Drawing for the job (mm, zero at the part's lowest x, y, z). A direction names the side the tool comes from. Round coordinates to 2 decimals unless told otherwise and drop trailing zeros. Loops run counter-clockwise (first coordinate to the right, second up) from the corner with the lowest first, then second, coordinate; pieces in that order, holes last. Notation, with made-up numbers: M -14.5,16.5 L 41.5,16.5 A25 cw 41.5,51.5 Z; hole C 6,15.5 d10. An arc over 180 degrees is marked long. Use a Markdown table: item, result. Add a question column.
Q1. Mould opens along Y. For the marked faces 1, 2, 3 and 4 say: +Y half, -Y half, draft (parallel to the pull), parting line (faces both ways), or undercut.
Q2. Cut at C-C (y = 18.5). Give the cut face in (x, z).
Q3. Probe line 1 (Y direction, x = 6.85, z = 0.6); line 2 (Z direction, x = 3, y = 13); line 3 (Z direction, x = 13, y = 24). List the from-to ranges inside material, lowest first. Write a range as from..to.
Q4. Tool access for the marked faces 5, 6 and 7: list every direction of +Z, -Z, +X, -X, +Y, -Y with a clear straight run to the whole face (end or side of a thin tool).
Q5. Cut at D-D (x = 11.25). Give the cut face in (y, z).
Q6. Pin check, flat tips, straight feed: pin 1 (2.5 mm diameter, centred on x = 6.85, y = 10.025, fed in from +Z); pin 2 (2 mm diameter, centred on y = 7, z = 7, fed in from +X); pin 3 (3 mm diameter, centred on x = 9, z = 5.5, fed in from +Y); pin 4 (4.5 mm diameter, centred on y = 20, z = 5.5, fed in from -X). Stop position of each tip, or through.
Q7. Cut at B-B (z = 5.75). Give the cut face in (x, y).
Q8. Cut at A-A (x = 6.85). Give the cut face in (y, z).
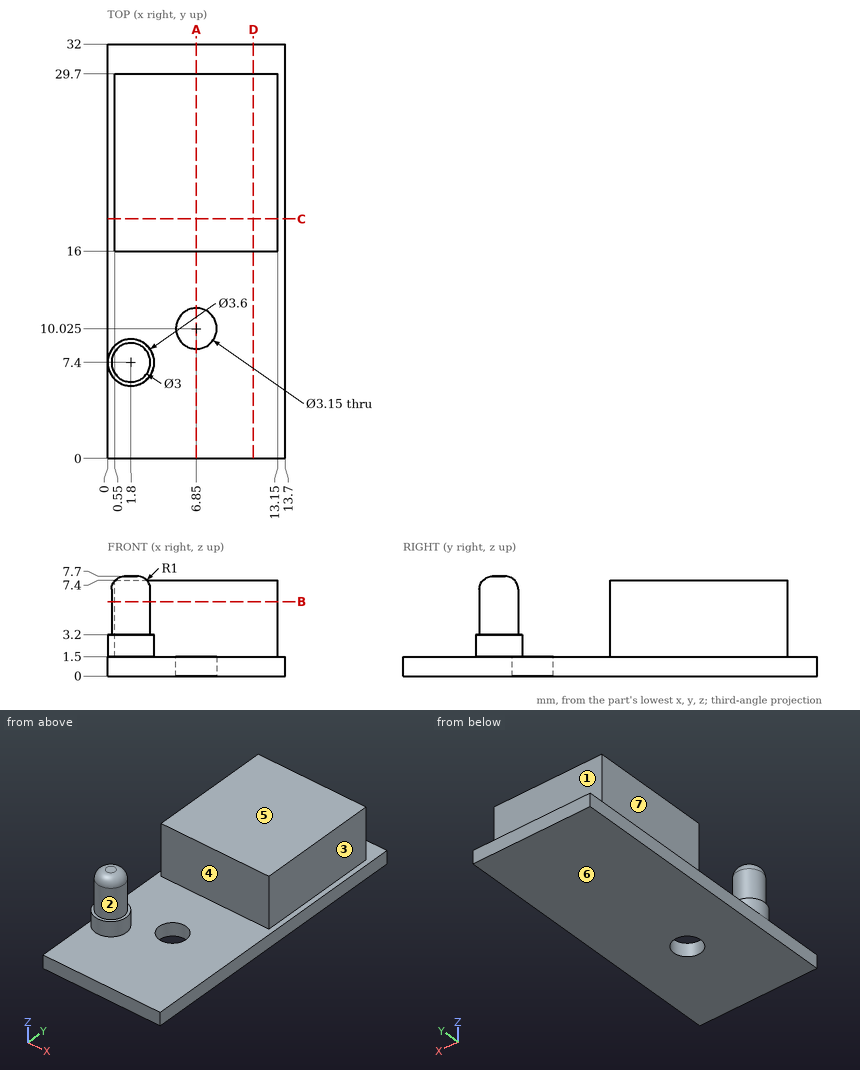
Checked values:
| question | item | result |
|---|---|---|
| 1 | face 1 | +Y half |
| 1 | face 2 | undercut |
| 1 | face 3 | draft |
| 1 | face 4 | undercut |
| 2 | outline | M 0,0 L 13.7,0 L 13.7,1.5 L 13.15,1.5 L 13.15,7.4 L 0.55,7.4 L 0.55,1.5 L 0,1.5 Z |
| 3 | line 1 | y = 0..8.45, 11.6..32 |
| 3 | line 2 | z = 0..1.5 |
| 3 | line 3 | z = 0..7.4 |
| 4 | face 5 | +Z, +X, -X, +Y |
| 4 | face 6 | -Z, +X, -X, +Y, -Y |
| 4 | face 7 | +Z, -X, +Y |
| 5 | outline | M 0,0 L 32,0 L 32,1.5 L 29.7,1.5 L 29.7,7.4 L 16,7.4 L 16,1.5 L 0,1.5 Z |
| 6 | pin 1 | passes through |
| 6 | pin 2 | stops at x = 3.3 |
| 6 | pin 3 | stops at y = 29.7 |
| 6 | pin 4 | stops at x = 0.55 |
| 7 | outline | C 1.8,7.4 d3; M 0.55,16 L 13.15,16 L 13.15,29.7 L 0.55,29.7 Z |
| 8 | outline | M 0,0 L 8.45,0 L 8.45,1.5 L 0,1.5 Z; M 11.6,0 L 32,0 L 32,1.5 L 29.7,1.5 L 29.7,7.4 L 16,7.4 L 16,1.5 L 11.6,1.5 Z |
